Read the model definition and answer for the solid it produces. Units are mm, in the model's axes. A direction names the side the tool comes from. Round coordinates to 2 decimals unless told otherwise and drop trailing zeros. Order: outer loops, then holes, each group sorted by start corner. A loop starts at its lowest first (then second) coordinate and runs counter-clockwise, first axis right, second up. Notation, with made-up numbers: (-12, -40) - (43, -40) arc R35 cw to (43, -1) - close; hole circle Ø11 at (-37, -38). An arc over 180 degrees is marked (long way). One line per question, with ' | ' between items. Start each with the question number.
1) Straight lines are drawn through the part: line 1 (Z direction, x = 30.75, y = 10); line 2 (Y direction, x = -32.25, z = -13.5); line 3 (Z direction, x = -32, y = 9.5). For each, find the intervals that lie inside material, in ascending order. Write a range as from..to.
2) The part is cut by section B-B, the plane x = 34. Give the vertices of the cut face in (y, z).
3) The part is cut by section D-D, the plane y = 2.25. Give the vertices of the cut face in (x, z).
4) The part is cut by section C-C, the plane x = 19. Give the vertices of the cut face in (y, z) (3 decimals).
5) Flat-ended cylindrical pins translate along their axes: pin 1 (1.5 mm diameter, centred on y = 9.5, z = -12.5, fed in from +X); pin 2 (10 mm diameter, centred on x = -4, y = 7.5, fed in from +Z); pin 3 (12 mm diameter, centred on x = 11, y = 16, fed in from +Z); pin 4 (6.5 mm diameter, centred on y = 10, z = 18.72, fed in from +X). Find the tip coordinate at first contact, or state that the pin passes through.
6) The mould has two halves that part along Z. Classify faces 5 (the flat face through (-1, 20, -4)), 6 (the cylindrical face through (-32.84, 11.95, 24.92)), 7 (the flat face through (-1, 10, -22.721)): pulls with the +Z half, pulls with the -Z half, needs draft (parallel to the pull), parting line crosses it, or undercut.
7) The part is cut by section A-A, the plane z = 10. Give the vertices of the cut face in (x, y).
8) For faces 1 (the flat face through (17.5, 12, 15)), 2 (the cylindrical face through (31, 12, -15)), 3 (the flat face through (-39, 10, 3)), 4 (the flat face through (-29, 10, 6)), determine the directions among +Z, -Z, +X, -X, +Y, -Y from which every point of the face is accessible in a straight line to the end or side of a thin tool.
from build123d import *

# Parameters (mm, degrees)
SKETCH_1_W           = 78
SKETCH_1_H           = 54.441624366
EXTRUDE_1_DEPTH      = 20
CUT_EXTRUDE_1_DEPTH  = 52.59430798
SKETCH_3_R           = 2.5
CUT_EXTRUDE_2_DEPTH  = 15
SKETCH_4_R           = 2.1
CUT_EXTRUDE_3_DEPTH  = 10
SKETCH_5_R           = 6.5
CUT_EXTRUDE_4_DEPTH  = 12.5
SKETCH_6_R           = 4.025
CUT_EXTRUDE_5_DEPTH  = 74.696829076
CUT_EXTRUDE_START    = -12.5
SKETCH_7_R           = 6.5
CUT_EXTRUDE_6_DEPTH  = 12.5
CUT_EXTRUDE_START_2  = -15
SKETCH_11_R          = 2.5
CUT_EXTRUDE_9_DEPTH  = 15
CUT_EXTRUDE_START_3  = -10
SKETCH_12_R          = 2.1
CUT_EXTRUDE_10_DEPTH = 10
SKETCH_9_W           = 4.5
SKETCH_9_H           = 20
CUT_EXTRUDE_8_DEPTH  = 85.999838917
CHAMFER_3_SIZE       = 0.5


with BuildPart() as part:
    # 草图1 → 凸台-拉伸1 (new body)
    with BuildSketch(Plane(origin=(0, 0, 0), x_dir=(1, 0, 0), z_dir=(0, 1, 0))):
        Rectangle(SKETCH_1_W, SKETCH_1_H)
    extrude(amount=EXTRUDE_1_DEPTH)

    # 草图2 → 切除-拉伸1 (cut, through all)
    with BuildSketch(Plane(origin=(0, 20, 0), x_dir=(1, 0, 0), z_dir=(0, 1, 0))):
        with BuildLine():
            Line((-17.5, -27.220812183), (17.5, -27.220812183))
            Line((17.5, -27.220812183), (17.5, -2.220812183))
            ThreePointArc((17.5, -2.220812183), (16.035533906, 1.314721723), (12.5, 2.779187817))
            Line((12.5, 2.779187817), (-12.5, 2.779187817))
            ThreePointArc((-12.5, 2.779187817), (-16.035533906, 1.314721723), (-17.5, -2.220812183))
            Line((-17.5, -2.220812183), (-17.5, -27.220812183))
        make_face()
    extrude(amount=-CUT_EXTRUDE_1_DEPTH, mode=Mode.SUBTRACT)

    # 草图3 → 切除-拉伸2 (cut)
    with BuildSketch(Plane.ZY.offset(39)):
        with Locations((-13.5, 10)):
            Circle(SKETCH_3_R)
    extrude(amount=-CUT_EXTRUDE_2_DEPTH, mode=Mode.SUBTRACT)

    # 草图4 → 切除-拉伸3 (cut)
    with BuildSketch(Plane.ZY.offset(39)):
        with Locations((6, 10)):
            Circle(SKETCH_4_R)
    extrude(amount=-CUT_EXTRUDE_3_DEPTH, mode=Mode.SUBTRACT)

    # 草图5 → 切除-拉伸4 (cut)
    with BuildSketch(Plane.ZY.offset(39)):
        with Locations((18.720812183, 10)):
            Circle(SKETCH_5_R)
    extrude(amount=-CUT_EXTRUDE_4_DEPTH, mode=Mode.SUBTRACT)

    # 草图6 → 切除-拉伸5 (cut, through all)
    with BuildSketch(Plane.ZY.offset(26.5)):
        with Locations((18.720812183, 10)):
            Circle(SKETCH_6_R)
    extrude(amount=-CUT_EXTRUDE_5_DEPTH, mode=Mode.SUBTRACT)

    # 草图7 → 切除-拉伸6 (cut)
    with BuildSketch(Plane(origin=(39, 0, 0), x_dir=(0, 0, -1), z_dir=(1, 0, 0)).offset(CUT_EXTRUDE_START)):
        with Locations(Location((-18.720812183, 10, 0), (0, 0, 180))):
            Circle(SKETCH_7_R)
    extrude(amount=CUT_EXTRUDE_6_DEPTH, mode=Mode.SUBTRACT)

    # 草图11 → 切除-拉伸9 (cut)
    with BuildSketch(Plane(origin=(39, 0, 0), x_dir=(0, 0, -1), z_dir=(1, 0, 0)).offset(CUT_EXTRUDE_START_2)):
        with Locations(Location((13.5, 10, 0), (0, 0, 180))):
            Circle(SKETCH_11_R)
    extrude(amount=CUT_EXTRUDE_9_DEPTH, mode=Mode.SUBTRACT)

    # 草图12 → 切除-拉伸10 (cut)
    with BuildSketch(Plane(origin=(39, 0, 0), x_dir=(0, 0, -1), z_dir=(1, 0, 0)).offset(CUT_EXTRUDE_START_3)):
        with Locations(Location((-6, 10, 0), (0, 0, 180))):
            Circle(SKETCH_12_R)
    extrude(amount=CUT_EXTRUDE_10_DEPTH, mode=Mode.SUBTRACT)

    # 草图9 → 切除-拉伸8 (cut, through all)
    with BuildSketch(Plane.ZY.offset(39)):
        with Locations((-24.970812183, 10)):
            Rectangle(SKETCH_9_W, SKETCH_9_H)
    extrude(amount=-CUT_EXTRUDE_8_DEPTH, mode=Mode.SUBTRACT)

    # 倒角3
    chamfer_3_edges = [part.edges().sort_by_distance(p)[0] for p in [
        (28.25, 0, 27.220812183),
        (-28.25, 20, 27.220812183),
        (28.25, 20, 27.220812183),
        (-28.25, 0, 27.220812183),
        (0, 20, -22.720812183),
        (0, 0, -22.720812183),
    ]]
    chamfer(chamfer_3_edges, length=CHAMFER_3_SIZE)


solid = part.part
Values:
1) line 1: z = -22.72..-16, -11..3.9, 8.1..12.22, 25.22..27.22 | line 2: y = 0..7.5, 12.5..20 | line 3: z = -22.72..-15.95, -11.05..3.96, 8.04..12.24, 25.2..27.22
2) outline: (0, -22.22) - (0.5, -22.72) - (19.5, -22.72) - (20, -22.22) - (20, 26.72) - (19.5, 27.22) - (0.5, 27.22) - (0, 26.72) - close; hole circle Ø13 at (10, 18.72); hole circle Ø5 at (10, -13.5); hole circle Ø4.2 at (10, 6)
3) outline: (-39, -22.72) - (39, -22.72) - (39, 27.22) - (17.5, 27.22) - (17.5, 2.22) arc R5 cw to (12.5, -2.78) - (-12.5, -2.78) arc R5 cw to (-17.5, 2.22) - (-17.5, 27.22) - (-39, 27.22) - close
4) outline: (0, -22.221) - (0.5, -22.721) - (19.5, -22.721) - (20, -22.221) - (20, 26.721) - (19.5, 27.221) - (0.5, 27.221) - (0, 26.721) - close; hole circle Ø8.05 at (10, 18.721)
5) pin 1: stops at x = 24 | pin 2: stops at z = -2.78 | pin 3: stops at z = 0.04 | pin 4: passes through
6) face 5: needs draft | face 6: undercut | face 7: pulls with the -Z half
7) outline: (-39, 0) - (-17.5, 0) - (-17.5, 20) - (-39, 20) - close; (17.5, 0) - (39, 0) - (39, 20) - (17.5, 20) - close
8) face 1: +Z, +Y, -Y | face 2: +X | face 3: +Z, -Z, -X, +Y, -Y | face 4: -X
